Build history of the part. All positions in model axes, mm. Round coordinates to 2 decimals unless told otherwise and drop trailing zeros. Write each loop counter-clockwise with the first axis right and the second up, starting at its lowest first coordinate (ties: lowest second). Pieces come first, ordered by that corner, then holes.
Item 1: Wall check: probe 1 along X at (y, z) = (0.75, -7); probe 2 along Z at (x, y) = (-1, 1); probe 3 along Y at (x, z) = (2.5, 3.5). Give the ranges that are in metal, low to high.
Item 2: Drop flat-ended pins along their axis: pin 1 Ø1.5 at (x, y) = (5.5, -4.5) entering from -Z; pin 2 Ø2.5 at (x, z) = (0, 3.5) entering from +Y; pin 3 Ø1.5 at (y, z) = (-0.5, 12) entering from +X. Give the stop position or say it passes through.
Item 3: Band-saw the part on A-A, the plane y = -2.25. Write the cut outline in (x, z) (3 decimals), then the cut area to 3 significant figures.
Item 4: Band-saw the part on B-B, the plane y = -5. Write the cut outline in (x, z), then the cut area to 3 significant figures.
Item 5: Mould opens along Z. For faces 1 (the flat face through (0, -5.503, 0)), 2 (the flat face through (0, 1.27, 3)), 3 (the cylindrical face through (3.441, -2.087, -15.497)) say: +Z half, -Z half, draft (parallel to the pull), parting line (faces both ways), or undercut.
Autodesk Inventor part; units mm, degrees
ref_plane "YZ Plane" through (0, 0, 0) normal (1, 0, 0) x (0, 1, 0)
ref_plane "XZ Plane" through (0, 0, 0) normal (0, 1, 0) x (-1, 0, 0)
ref_plane "XY Plane" through (0, 0, 0) normal (0, 0, 1) x (1, 0, 0)
sketch "Sketch1" plane through (0, 0, 0) normal (0, 0, 1) x (1, 0, 0)
  line L0 (-15.875, 0) -> (0, 0)
  line L1 (0, 0) -> (0, -4.2333)
  line L2 (0, -4.2333) -> (-15.875, -4.2333)
  line L3 (-15.875, -4.2333) -> (-15.875, 0)
  line L4 (0, -4.2333) -> (-13.97, -4.2333)
  line L5 (-13.97, -4.2333) -> (-13.97, -5.5033)
  line L6 (-13.97, -5.5033) -> (0, -5.5033)
  line L7 (0, -5.5033) -> (0, -4.2333)
  line L8 (-15.875, -4.2333) -> (-13.6299, -4.2333) construction
  line L9 (-15.875, 0) -> (-12.7, 0) construction
  line L10 (-13.97, 1.27) -> (0, 1.27)
  line L11 (0, 1.27) -> (0, 0)
  line L12 (0, 0) -> (-13.97, 0)
  line L13 (-13.97, 0) -> (-13.97, 1.27)
  line L14 (-15.875, 0) -> (-12.8362, 0) construction
  line L15 (-15.875, -4.2333) -> (-13.97, -5.5033)
  line L16 (-15.875, 0) -> (-14.9225, 1.905)
  line L17 (-14.9225, 1.905) -> (-13.97, 1.27)
  line L18 (-13.97, 0) -> (-15.875, 0)
  line L19 (0, -6.985) -> (0, 3.3867)
  point P0 (0, 0)
  point P1 (-13.97, 0.635)
  point P2 (0, 0.635)
  point P3 (-6.985, -4.2333)
  point P4 (-14.9225, 0)
  dimension "d0" = 0
  dimension "d1" = 4.2333
  dimension "d2" = 15.875
  dimension "d3" = 0
  dimension "d5" = 13.97
  dimension "d9" = 13.97
  dimension "d10" = 1.27
  dimension "d11" = 1.27
  dimension "d12" = 0.635
  dimension "d13" = 0
revolve "Revolution1" add sketch "Sketch1" angle 360 about axis through (0, -10, 0) along (0, 1, 0)
sketch "Sketch2" plane through (0, 1.27, 0) normal (0, 1, 0) x (1, 0, 0)
  line L0 (-2.3268, -5.2364) -> (-2.3268, -8.072)
  line L1 (-2.3268, -8.072) -> (-0.6076, -8.072)
  line L2 (-0.6076, -8.072) -> (-0.6076, -5.355)
  line L3 (-0.6076, -5.355) -> (0.1136, -5.355)
  line L4 (0.1136, -5.355) -> (0.1136, -8.072)
  line L5 (0.1136, -8.072) -> (3.048, -8.072)
  line L6 (3.048, -8.072) -> (3.048, -8.8822)
  line L7 (3.048, -8.8822) -> (-3.048, -8.8822)
  line L8 (-3.048, -8.8822) -> (-3.048, -5.2364)
  line L9 (-3.048, -5.2364) -> (-2.3268, -5.2364)
  line L10 (3.048, -5.1673) -> (-3.048, -3.1122)
  line L11 (-3.048, -3.1122) -> (-3.048, -2.1143)
  line L12 (-3.048, -2.1143) -> (3.048, -0.0593)
  line L13 (3.048, -0.0593) -> (3.048, -0.9139)
  line L14 (3.048, -0.9139) -> (1.3437, -1.4672)
  line L15 (1.3437, -1.4672) -> (1.3437, -3.7939)
  line L16 (1.3437, -3.7939) -> (3.048, -4.3472)
  line L17 (3.048, -4.3472) -> (3.048, -5.1673)
  line L18 (0.6521, -1.6895) -> (-2.2181, -2.633)
  line L19 (-2.2181, -2.633) -> (0.6521, -3.5716)
  line L20 (0.6521, -3.5716) -> (0.6521, -1.6895)
  line L21 (3.048, 1.9414) -> (-2.3268, 1.9414)
  line L22 (-2.3268, 1.9414) -> (-2.3268, -0.1037)
  line L23 (-2.3268, -0.1037) -> (-3.048, -0.1037)
  line L24 (-3.048, -0.1037) -> (-3.048, 4.7968)
  line L25 (-3.048, 4.7968) -> (-2.3268, 4.7968)
  line L26 (-2.3268, 4.7968) -> (-2.3268, 2.7516)
  line L27 (-2.3268, 2.7516) -> (3.048, 2.7516)
  line L28 (3.048, 2.7516) -> (3.048, 1.9414)
  line L29 (3.048, 5.4143) -> (-3.048, 5.4143)
  line L30 (-3.048, 5.4143) -> (-3.048, 9.228)
  line L31 (-3.048, 9.228) -> (-2.3268, 9.228)
  line L32 (-2.3268, 9.228) -> (-2.3268, 6.2244)
  line L33 (-2.3268, 6.2244) -> (-0.657, 6.2244)
  line L34 (-0.657, 6.2244) -> (-0.657, 9.0254)
  line L35 (-0.657, 9.0254) -> (0.0642, 9.0254)
  line L36 (0.0642, 9.0254) -> (0.0642, 6.2244)
  line L37 (0.0642, 6.2244) -> (2.3268, 6.2244)
  line L38 (2.3268, 6.2244) -> (2.3268, 9.228)
  line L39 (2.3268, 9.228) -> (3.048, 9.228)
  line L40 (3.048, 9.228) -> (3.048, 5.4143)
  point P0 (0, 0)
  point P1 (0, 0)
extrude "Extrusion1" cut sketch "Sketch2" against normal blind 0.7937
equation "\"d17\" = 0.5 * d16"
properties part number "Fate Game Piece V1.01"
Results:
1. probe 1: x = -13.83 to -3.05, -2.33 to -0.66, 0.06 to 2.33, 3.05 to 13.83
1. probe 2: z = -15.34 to -6.22, -5.41 to -2.75, -1.94 to 1.42, 2.23 to 3.03, 3.8 to 8.07, 8.88 to 15.34
1. probe 3: y = -5.5 to 1.27
2. pin 1: stops at z = -15.13
2. pin 2: stops at y = 1.27
2. pin 3: stops at x = 11.2
3. outline: circle Ø31.75 at (0, 0)
3. area: 792 mm2
4. outline: circle Ø29.45 at (0, 0)
4. area: 681 mm2
5. face 1: draft
5. face 2: undercut
5. face 3: parting line
